from build123d import *

# Parameters (mm, degrees)
F0_R     = 75
F0_R_2   = 65
F0_R_3   = 51
F1_DEPTH = 30
F3_DEPTH = 12
F4_R     = 5
F5_R     = 15
F6_DEPTH = 15
F7_DEPTH = 12.5


with BuildPart() as f1:
    # F0 (on Top) → F1 (new body)
    with BuildSketch(Plane.XY):
        Circle(F0_R)
        Circle(F0_R_2, mode=Mode.SUBTRACT)
        Circle(F0_R_2)
        Circle(F0_R_3, mode=Mode.SUBTRACT)
    extrude(amount=F1_DEPTH)

    # F0 (on Top) → F3 (cut)
    with BuildSketch(Plane.XY):
        Circle(F0_R_2)
        Circle(F0_R_3, mode=Mode.SUBTRACT)
    extrude(amount=F3_DEPTH, mode=Mode.SUBTRACT)

    # F4
    f4_edges = [f1.edges().sort_by_distance(p)[0] for p in [
        (-65, 0, 12),
    ]]
    fillet(f4_edges, radius=F4_R)

    # F5
    f5_edges = [f1.edges().sort_by_distance(p)[0] for p in [
        (-75, 0, 30),
    ]]
    fillet(f5_edges, radius=F5_R)

    # F2 (on face) → F6 (cut)
    with BuildSketch(Plane.XY.offset(30)):
        with BuildLine():
            Line((52.6, -2), (74.9733285909, -2))
            ThreePointArc((74.9733285909, -2), (74.9933318513, -1.0000889166), (75, 0))
            ThreePointArc((75, 0), (74.9933318513, 1.0000889166), (74.9733285909, 2))
            Line((74.9733285909, 2), (52.6, 2))
            Line((52.6, 2), (52.6, -2))
        make_face()
        with BuildLine():
            Line((52.6, 2), (74.9733285909, 2))
            ThreePointArc((74.9733285909, 2), (74.8492284695, 4.7532091816), (74.624057783, 7.5))
            Line((74.624057783, 7.5), (52.6, 7.5))
            Line((52.6, 7.5), (52.6, 2))
        make_face()
        with BuildLine():
            ThreePointArc((74.624057783, -7.5), (74.8492284695, -4.7532091816), (74.9733285909, -2))
            Line((74.9733285909, -2), (52.6, -2))
            Line((52.6, -2), (52.6, -7.5))
            Line((52.6, -7.5), (74.624057783, -7.5))
        make_face()
        with BuildLine():
            Line((-52.6, 7.5), (-74.624057783, 7.5))
            ThreePointArc((-74.624057783, 7.5), (-74.8492284695, 4.7532091816), (-74.9733285909, 2))
            Line((-74.9733285909, 2), (-52.6, 2))
            Line((-52.6, 2), (-52.6, 7.5))
        make_face()
        with BuildLine():
            ThreePointArc((-75, 0), (-74.9933318513, -1.0000889166), (-74.9733285909, -2))
            Line((-74.9733285909, -2), (-52.6, -2))
            Line((-52.6, -2), (-52.6, 2))
            Line((-52.6, 2), (-74.9733285909, 2))
            ThreePointArc((-74.9733285909, 2), (-74.9933318513, 1.0000889166), (-75, 0))
        make_face()
        with BuildLine():
            ThreePointArc((-74.9733285909, -2), (-74.8492284695, -4.7532091816), (-74.624057783, -7.5))
            Line((-74.624057783, -7.5), (-52.6, -7.5))
            Line((-52.6, -7.5), (-52.6, -2))
            Line((-52.6, -2), (-74.9733285909, -2))
        make_face()
    extrude(amount=-F6_DEPTH, mode=Mode.SUBTRACT)

    # F2 (on face) → F7 (cut)
    with BuildSketch(Plane.XY.offset(30)):
        with BuildLine():
            Line((-52.6, -2), (-50.960769225, -2))
            ThreePointArc((-50.960769225, -2), (-51, 0), (-50.960769225, 2))
            Line((-50.960769225, 2), (-52.6, 2))
            Line((-52.6, 2), (-52.6, -2))
        make_face()
        with BuildLine():
            Line((50.960769225, -2), (52.6, -2))
            Line((52.6, -2), (52.6, 2))
            Line((52.6, 2), (50.960769225, 2))
            ThreePointArc((50.960769225, 2), (50.990191363, 1.0001923632), (51, 0))
            ThreePointArc((51, 0), (50.990191363, -1.0001923632), (50.960769225, -2))
        make_face()
    extrude(amount=-F7_DEPTH, mode=Mode.SUBTRACT)


solid = f1.part
CAD build for the part. Positions are in the model's coordinates, mm. A direction names the side the tool comes from. Give positions to 0.01 mm unless a question says otherwise; leave off trailing zeros. Write each loop counter-clockwise with the first axis right and the second up, starting at its lowest first coordinate (ties: lowest second). Pieces come first, ordered by that corner, then holes. Notation, with made-up numbers: (20, 28) - (39, 28) arc R32 cw to (39, 65) - close; hole circle Ø8 at (65, 46.5). An arc over 180 degrees is marked (long way). Put each result on its own line as item: value.
(1) Pull direction X, two halves, no side cores. Call faces 1 (the flat face through (61, 7.5, 23)), 2 (the flat face through (52.6, 3, 23)), 3 (the cylindrical face through (62, 19.52, 3.45)): released by +X, released by -X, zero draft, split by the parting line, or undercut.
Working result:
face 1: zero draft
face 2: released by +X
face 3: undercut
(2) Saw through at B-B (y = 0). List the corners of the cut face in (x, z), then the cut area to 3 significant figures.
Working result:
outline: (-75, 0) - (-65, 0) - (-65, 7) arc R5 cw to (-60, 12) - (-51, 12) - (-51, 17.5) - (-52.6, 17.5) - (-52.6, 15) - (-75, 15) - close; (51, 12) - (60, 12) arc R5 cw to (65, 7) - (65, 0) - (75, 0) - (75, 15) - (52.6, 15) - (52.6, 17.5) - (51, 17.5) - close
area: 403 mm^2
(3) Saw through at D-D (z = 5). List the corners of the cut face in (x, y), then the cut area to 3 significant figures.
Working result:
outline: circle Ø150 at (0, 0); hole circle Ø130 at (0, 0)
area: 4,400 mm^2
(4) Tool access for faces 4 (the flat face through (64, 0, 15)), 5 (the flat face through (-27, -44, 12)), 6 (the flat face through (-64, 0, 15)): list every direction of +Z, -Z, +X, -X, +Y, -Y with a clear straight run to the whole face (end or side of a thin tool).
Working result:
face 4: +Z, +X
face 5: -Z
face 6: +Z, -X
(5) Drop flat-ended pins along their axis: pin 1 Ø12 at (y, z) = (-0.5, 24.5) entering from -X; pin 2 Ø6 at (y, z) = (-7, 17) entering from -X; pin 3 Ø12 at (x, y) = (69, 3) entering from +Z. Give the stop position or say it passes through.
Working result:
pin 1: x = -52.6
pin 2: x = -74.85
pin 3: z = 28.97
(6) Saw through at A-A (x = 0). List the corners of the cut face in (y, z).
Working result:
outline: (-75, 0) - (-65, 0) - (-65, 7) arc R5 cw to (-60, 12) - (-51, 12) - (-51, 30) - (-60, 30) arc R15 ccw to (-75, 15) - close; (51, 12) - (60, 12) arc R5 cw to (65, 7) - (65, 0) - (75, 0) - (75, 15) arc R15 ccw to (60, 30) - (51, 30) - close
(7) Wall check: L1, parallel to Z at x = 35, y = 45; L2, parallel to Y at x = -10.5, z = 28; L3, parallel to X at y = -43, z = 6.5. Give the ranges that are in metal, low to high.
Working result:
L1: 12 to 30
L2: -66.66 to -49.91, 49.91 to 66.66
L3: -61.45 to -48.74, 48.74 to 61.45
(8) Saw through at C-C (z = 20.5). List the corners of the cut face in (x, y), then the cut area to 3 significant figures.
Working result:
outline: (-73.57, -7.5) arc R73.96 ccw to (73.57, -7.5) - (52.6, -7.5) - (52.6, -2) - (50.96, -2) arc R51 cw to (-50.96, -2) - (-52.6, -2) - (-52.6, -7.5) - close; (-73.57, 7.5) - (-52.6, 7.5) - (-52.6, 2) - (-50.96, 2) arc R51 cw to (50.96, 2) - (52.6, 2) - (52.6, 7.5) - (73.57, 7.5) arc R73.96 ccw to start
area: 8,360 mm^2
